The listing builds one solid part. Answer for the finished solid, in the listing's coordinates (mm). A direction names the side the tool comes from. Give positions to 0.01 mm unless a question says otherwise; leave off trailing zeros. Order: outer loops, then holes, each group sorted by start corner. A loop starts at its lowest first (then second) coordinate and runs counter-clockwise, first axis right, second up. Notation, with made-up numbers: (-5.75, 3) - (14.25, 3) arc R17 ccw to (14.25, 33) - close; hole circle Ø3 at (-21.5, 27). An arc over 180 degrees is marked (long way). Answer as a JSON object with one key per item and string values. Group by question number.
Q1. The mould has two halves that part along Y. Classify faces 3 (the face through (1.34, -2.11, -52.28)), 4 (the face through (4.908, -1.546, -76.3)), 5 (the face through (-3, -6, -104.775)), 6 (the face through (3.399, 6.535, -103.081)): released by +Y, released by -Y, zero draft, split by the parting line, or undercut.
Q2. Given pin 1 (1 mm diameter, centred on y = 3, z = -67, fed in from +X); pin 2 (9 mm diameter, centred on x = -3, y = 0, fed in from -Z) (3 decimals); pin 3 (1.5 mm diameter, centred on y = 3.5, z = -92.5, fed in from -X); pin 4 (3 mm diameter, centred on x = 6, z = -77.5, fed in from -Y), each flat-ended and moving along its own axis, determine where each tip first touches the part or whether it passes through.
Q3. Consider line 1 (Y direction, x = 0, z = -59.05); line 2 (X direction, y = 1.5, z = -77); line 3 (X direction, y = 0.75, z = -55.5). Determine where each line is inside the solid, lowest interval first.
Q4. A cutting plane is placed at C-C, the plane z = -87. Give the vertices of the cut face in (x, y), and give its area (3 significant figures).
Q5. A cutting plane is placed at D-D, the plane z = -71. Give the vertices of the cut face in (x, y), and give its area (3 significant figures).
Q6. For faces 1 (the face through (0.124, 6.193, -70.792)), 2 (the face through (-5.04, 3.86, -98.34)), determine the directions among +Z, -Z, +X, -X, +Y, -Y from which every point of the face is accessible in a straight line to the end or side of a thin tool.
from build123d import *

# Parameters (mm, degrees)
SKETCH11_W                     = 36.563301826
SKETCH11_H                     = 1.5875
FILLET1_R                      = 0.254
CE_00_MILL_ONE_SIDE_FLAT_DEPTH = 12.7
CP_00_MILL_PATTERN_COUNT       = 4
FILLET2_R                      = 0.0508


with BuildPart() as part:
    # Sketch17 → BR-00 Lathe Initial (revolve)
    with BuildSketch(Plane(origin=(0, 0, 0), x_dir=(0, 0, -1), z_dir=(1, 0, 0)), mode=Mode.PRIVATE) as br_00_lathe_initial_sk:
        Polygon((105.41, 15.875), (105.41, 0), (17.129076381, 0), (17.129076381, 2.163905573), (40.590225916, 5.127738011), (40.590225916, 8.7376), (69.165225916, 8.7376), (69.165225916, 15.875), align=None)
    revolve(br_00_lathe_initial_sk.sketch.rotate(Axis((0, 0, -105.41), (0, 0, -1)), 180), axis=Axis((0, 0, -105.41), (0, 0, -1)))

    # Sketch11 → CR-00 Bore at tip (revolve, cut)
    with BuildSketch(Plane(origin=(0, 0, 0), x_dir=(0, 0, -1), z_dir=(1, 0, 0)), mode=Mode.PRIVATE) as cr_00_bore_at_tip_sk:
        with Locations((34.401809356, 0.79375)):
            Rectangle(SKETCH11_W, SKETCH11_H)
    revolve(cr_00_bore_at_tip_sk.sketch.rotate(Axis((0, 0, 50), (0, 0, -1)), 90), axis=Axis((0, 0, 50), (0, 0, -1)), mode=Mode.SUBTRACT)

    # Sketch16 → CR-00 Lathe at tip (revolve, cut)
    with BuildSketch(Plane(origin=(0, 0, 0), x_dir=(0, 0, -1), z_dir=(1, 0, 0)), mode=Mode.PRIVATE) as cr_00_lathe_at_tip_sk:
        with BuildLine():
            Line((15.596764062, 0.762), (17.637076381, 0.762))
            Line((17.637076381, 0.762), (20.471990781, 0.762))
            Line((20.471990781, 0.762), (20.471990781, 1.5875))
            Line((20.471990781, 1.5875), (19.959663009, 1.5875))
            Line((19.959663009, 1.5875), (19.959663009, 1.7399))
            Line((19.959663009, 1.7399), (20.848663009, 1.817677422))
            ThreePointArc((20.848663009, 1.817677422), (21.077336093, 1.895301474), (21.244328797, 2.069744329))
            Line((21.244328797, 2.069744329), (26.498763841, 11.17069279))
            Line((26.498763841, 11.17069279), (15.596764062, 11.17069279))
            Line((15.596764062, 11.17069279), (15.596764062, 0.762))
        make_face()
    revolve(cr_00_lathe_at_tip_sk.sketch.rotate(Axis((0, 0, -16.467430566), (0, 0, 1)), 90), axis=Axis((0, 0, -16.467430566), (0, 0, 1)), mode=Mode.SUBTRACT)

    # Sketch7 → CR-00 Bore form base ( flip around ) (revolve, cut)
    with BuildSketch(Plane(origin=(0, 0, 0), x_dir=(0, 0, -1), z_dir=(1, 0, 0)), mode=Mode.PRIVATE) as cr_00_bore_form_base_flip_around_sk:
        Polygon((42.949724835, 0), (137.038186875, 0), (137.038186875, 20.32), (101.6, 20.32), (101.6, 7.366), (104.775, 7.366), (104.775, 6.35), (92.075, 6.35), (60.96, 3.9751), (57.785, 3.9751), align=None)
    revolve(cr_00_bore_form_base_flip_around_sk.sketch.rotate(Axis((0, 0, -137.038186875), (0, 0, -1)), 90), axis=Axis((0, 0, -137.038186875), (0, 0, -1)), mode=Mode.SUBTRACT)

    # Sketch20 → CR-00 Lathe Next (revolve, cut)
    with BuildSketch(Plane(origin=(0, 0, 0), x_dir=(0, 0, -1), z_dir=(1, 0, 0)), mode=Mode.PRIVATE) as cr_00_lathe_next_sk:
        with BuildLine():
            Line((105.41, 13.316379782), (69.165225916, 8.7376))
            ThreePointArc((69.165225916, 8.7376), (68.56580235, 8.922006767), (68.307721992, 9.493591402))
            Line((68.307721992, 9.493591402), (68.307721992, 30.289247764))
            Line((68.307721992, 30.289247764), (105.41, 30.289247764))
            Line((105.41, 30.289247764), (105.41, 13.316379782))
        make_face()
    revolve(cr_00_lathe_next_sk.sketch.rotate(Axis((0, 0, -113.533763994), (0, 0, -1)), 270), axis=Axis((0, 0, -113.533763994), (0, 0, -1)), mode=Mode.SUBTRACT)

    # Fillet1
    fillet1_edges = [part.edges().sort_by_distance(p)[0] for p in [
        (-7.366, 0, -104.775),
    ]]
    fillet(fillet1_edges, radius=FILLET1_R)

    # Sketch18 → CE-00 Mill one side flat (cut, symmetric)
    with BuildSketch(Plane(origin=(0, 0, 0), x_dir=(0, 0, -1), z_dir=(1, 0, 0))):
        Polygon((125.778198054, 11.004166448), (12.733631993, 1.114048445), (12.733631993, 41.952542689), (125.778198054, 41.952542689), align=None)
    ce_00_mill_one_side_flat = extrude(amount=CE_00_MILL_ONE_SIDE_FLAT_DEPTH, both=True, mode=Mode.SUBTRACT)

    # CP-00 Mill pattern: CE-00 Mill one side flat ×4 about axis
    cp_00_mill_pattern_axis = Axis((0, 0, 0), (0, 0, 1))
    for i in range(1, CP_00_MILL_PATTERN_COUNT):
        add(ce_00_mill_one_side_flat.rotate(cp_00_mill_pattern_axis, i * 360 / CP_00_MILL_PATTERN_COUNT), mode=Mode.SUBTRACT)

    # Fillet2
    fillet2_edges = [part.edges().sort_by_distance(p)[0] for p in [
        (1.7399, 0, -19.959663009),
    ]]
    fillet(fillet2_edges, radius=FILLET2_R)


solid = part.part
Reply:
{
 "1": {"face 3": "undercut", "face 4": "undercut", "face 5": "zero draft", "face 6": "split by the parting line"},
 "2": {"pin 1": "stops at x = 5.91", "pin 2": "stops at z = -104.775", "pin 3": "stops at x = -8.16", "pin 4": "stops at y = -6.91"},
 "3": {"line 1": "y = -5.17 to -3.98, 3.98 to 5.17", "line 2": "x = -6.74 to -4.98, 4.98 to 6.74", "line 3": "x = -4.86 to -3.28, 3.28 to 4.86"},
 "4": {"outline": "(-7.61, -7.61) - (7.61, -7.61) - (7.61, 7.61) - (-7.61, 7.61) - close; hole circle Ø11.93 at (0, 0)", "area": "120 mm^2"},
 "5": {"outline": "(-6.21, -6.21) - (6.21, -6.21) - (6.21, 6.21) - (-6.21, 6.21) - close; hole circle Ø9.48 at (0, 0)", "area": "83.7 mm^2"},
 "6": {"face 1": "+Z, +X, -X, +Y", "face 2": "-Z"}
}
